```python
from build123d import *

# Parameters (mm, degrees)
SKETCH1_R           = 30.475
BOSS_EXTRUDE1_DEPTH = 130
SKETCH2_R           = 47.05874864
BOSS_EXTRUDE2_DEPTH = 20
SKETCH8_R           = 20
CUT_EXTRUDE1_DEPTH  = 40


with BuildPart() as part:
    # Sketch1 → Boss-Extrude1 (new body)
    with BuildSketch(Plane.XY):
        Circle(SKETCH1_R)
    extrude(amount=BOSS_EXTRUDE1_DEPTH)

    # Sketch2 → Boss-Extrude2 (add, symmetric)
    with BuildSketch(Plane(origin=(0, 0, 0), x_dir=(1, 0, 0), z_dir=(0, 1, 0))):
        with Locations((0, 35.858056257)):
            Circle(SKETCH2_R)
    extrude(amount=BOSS_EXTRUDE2_DEPTH, both=True)

    # Sketch8 → Cut-Extrude1 (cut)
    with BuildSketch(Plane(origin=(0, 20, 0), x_dir=(1, 0, 0), z_dir=(0, 1, 0))):
        with Locations(Location((0, 35.858056257, 0), (0, 0, 270))):
            Circle(SKETCH8_R)
    extrude(amount=-CUT_EXTRUDE1_DEPTH, mode=Mode.SUBTRACT)


solid = part.part
```
Build history of the part. All positions in model axes, mm. A direction names the side the tool comes from. Give positions to 0.01 mm unless a question says otherwise; leave off trailing zeros. Loops run counter-clockwise (first coordinate to the right, second up) from the corner with the lowest first, then second, coordinate; pieces in that order, holes last. Notation, with made-up numbers: (50, 40) -> (87, 40) arc R12 ccw to (87, 53) -> close; hole circle Ø7 at (-15, 25.5). An arc over 180 degrees is marked (long way). One line per question, with ' | ' between items. Start each with the question number.
1) Cut at C-C (y = 0). Give the cut face in (x, z) (1 decimal), plus the area to 3 significant figures.
2) Pin check, flat tips, straight feed: pin 1 (2 mm diameter, centred on x = 22, y = 10.5, fed in from -Z); pin 2 (8.5 mm diameter, centred on x = 2, y = -28, fed in from -Z); pin 3 (1 mm diameter, centred on y = -17, z = 57, fed in from -X). Stop position of each tip, or through.
3) Cut at D-D (x = -25.5). Give the cut face in (y, z).
4) 3-axis set-ups, long thin cutter, end or side, ignore diameter. For faces 5 (the flat face through (0, 24, 0)), 6 (the cylindrical face through (-3.967, 30.216, 64.088)): which of +Z, -Z, +X, -X, +Y, -Y reach the whole face in a straight line?
5) Cut at B-B (z = -34.5). Give the cut face in (x, y), plus the area to 3 significant figures.
6) Cut at A-A (x = 0). Give the cut face in (y, z) (3 decimals), plus the area to 3 significant figures.
7) Two-plate mould, pull along Z, no slides. Class faces 1 (the flat face through (0, -24, 0)), 2 (the flat face through (0, 0, 130)), 3 (the flat face through (20, 20, -39)), 4 (the cylindrical face through (6.007, 0.28, -16.782)): released by +Z, released by -Z, zero draft, split by the parting line, or undercut.
8) Probe L1, parallel to Z at x = -1, y = 5; L2, parallel to Z at x = -13.5, y = -26; L3, parallel to Y at x = 30.5, z = -38.5. List the from-to ranges inside material, lowest first.
Return value:
1) outline: (-30.5, 0) arc R47.1 ccw (long way) to (30.5, 0) -> (30.5, 130) -> (-30.5, 130) -> close; hole circle Ø40 at (0, -35.9) | area: 13,200 mm^2
2) pin 1: z = -77.97 | pin 2: z = 0 | pin 3: x = -25.62
3) outline: (-20, -75.41) -> (20, -75.41) -> (20, 3.69) -> (16.69, 3.69) -> (16.69, 130) -> (-16.69, 130) -> (-16.69, 3.69) -> (-20, 3.69) -> close
4) face 5: -Z, +X, -X, +Y | face 6: +Z
5) outline: (-47.04, -20) -> (-19.95, -20) -> (-19.95, 20) -> (-47.04, 20) -> close; (19.95, -20) -> (47.04, -20) -> (47.04, 20) -> (19.95, 20) -> close | area: 2,170 mm^2
6) outline: (-30.475, 0) -> (-20, 0) -> (-20, -15.858) -> (20, -15.858) -> (20, 0) -> (30.475, 0) -> (30.475, 130) -> (-30.475, 130) -> close; (-20, -82.917) -> (20, -82.917) -> (20, -55.858) -> (-20, -55.858) -> close | area: 9,640 mm^2
7) face 1: released by -Z | face 2: released by +Z | face 3: zero draft | face 4: undercut
8) L1: -82.91 to -55.83, -15.88 to 130 | L2: 0 to 130 | L3: -20 to 20
